Autodesk Inventor part; units mm, degrees
ref_plane "YZ Plane" through (0, 0, 0) normal (1, 0, 0) x (0, 1, 0)
ref_plane "XZ Plane" through (0, 0, 0) normal (0, 1, 0) x (-1, 0, 0)
ref_plane "XY Plane" through (0, 0, 0) normal (0, 0, 1) x (1, 0, 0)
sketch "Sketch1" plane through (0, 0, 0) normal (0, 1, 0) x (-1, 0, 0)
  circle A0 centre (0, 0) radius 9.625
  circle A1 centre (0, 0) radius 7.7
  dimension "d0" = 19.25
  dimension "d1" = 15.4
extrude "Extrusion1" add sketch "Sketch1" along normal blind 1
sketch "Sketch2" plane through (0, 1, 0) normal (0, 1, 0) x (1, 0, 0)
  circle A0 centre (0, 0) radius 9.6436
  line L0 (-2.8579, 4.95) -> (2.8579, 4.95)
  line L1 (2.8579, 4.95) -> (5.7158, 0)
  line L2 (5.7158, 0) -> (2.8579, -4.95)
  line L3 (2.8579, -4.95) -> (-2.8579, -4.95)
  line L4 (-2.8579, -4.95) -> (-5.7158, 0)
  line L5 (-5.7158, 0) -> (-2.8579, 4.95)
  line L6 (0, 0) -> (0, -3.104)
  line L7 (0, 0) -> (3.104, 0) construction
  dimension "d4" = 9.9
  dimension "d5" = 90
extrude "Extrusion2" add sketch "Sketch2" along normal blind 6
sketch "Sketch3" plane through (0, 7, 0) normal (0, 1, 0) x (1, 0, 0)
  circle A0 centre (0, 0) radius 9.6436
  circle A1 centre (0, 0) radius 2.75
  circle A2 centre (0, 0) radius 9.6436
  dimension "d8" = 5.5
  dimension "d9" = 0
extrude "Extrusion3" add sketch "Sketch3" along normal blind 1
fillet "Fillet1" radius 0.2 2 edges at (9.625, 0, 0) (7.7, 0, 0)
properties part number "NutRetainer"
Read the model definition and answer for the solid it produces. Units are mm, in the model's axes. A direction names the side the tool comes from. Give positions to 0.01 mm unless a question says otherwise; leave off trailing zeros. Loops run counter-clockwise (first coordinate to the right, second up) from the corner with the lowest first, then second, coordinate; pieces in that order, holes last. Notation, with made-up numbers: (-14.75, 77) - (-2.75, 77) arc R31 ccw to (-2.75, 102) - close; hole circle Ø4 at (74, -16.5). An arc over 180 degrees is marked (long way). Answer as CSV lines item,"result". Start each with the question number.
1) Which of the six approach directions +Z, -Z, +X, -X, +Y, -Y give full straight-line access (tool end or side, diameter ignored) to faces 5 (the face through (4.267, 3.958, -2.51)), 6 (the face through (-2.3, 8, 2))?
2) Find section B-B (y = 6). Write down the section's boundary in (x, z).
3) Determine the mould class of faces 1 (the face through (4.307, 3.958, 2.44)), 2 (the face through (0, 4, -4.95)), 3 (the face through (2, 0, -8)), 4 (the face through (7.638, 0.594, 5.857)) for opening direction Z: released by +Z, released by -Z, zero draft, split by the parting line, or undercut.
4) Each of these flat-tipped pins is pushed along its axis until it touches: pin 1 Ø3 at (x, y) = (-3, 2.5) entering from +Z; pin 2 Ø8 at (x, z) = (0, -0.5) entering from -Y; pin 3 Ø3 at (x, y) = (3, 2.5) entering from -Z; pin 4 Ø6.5 at (x, z) = (0, 0) entering from +Y. Where does it stop, or does it pass through?
5) Straight lines are drawn through the part: L1, parallel to X at y = 7.2, z = 0; L2, parallel to Z at x = 0, y = 0.85 (3 decimals). For each, find the intervals that lie inside material, in ascending order. Write a range as from..to.
6) Find section A-A (x = 0). Write down the section's boundary in (y, z) (3 decimals), then the cut area to 3 significant figures.
Findings below:
1,face 5,"-Y"
1,face 6,"+Z, -Z, +X, -X, +Y"
2,outline,"circle Ø19.29 at (0, 0); hole (-5.72, 0) - (-2.86, -4.95) - (2.86, -4.95) - (5.72, 0) - (2.86, 4.95) - (-2.86, 4.95) - close"
3,face 1,"undercut"
3,face 2,"undercut"
3,face 3,"zero draft"
3,face 4,"split by the parting line"
4,pin 1,"z = 9.53"
4,pin 2,"y = 7"
4,pin 3,"z = -9.53"
4,pin 4,"y = 8"
5,L1,"-9.64..-2.75, 2.75..9.64"
5,L2,"-9.625..-7.7, 7.7..9.625"
6,outline,"(0, -9.425) arc R0.2 ccw to (0.2, -9.625) - (1, -9.625) - (1, -9.644) - (8, -9.644) - (8, -2.75) - (7, -2.75) - (7, -4.95) - (1, -4.95) - (1, -7.7) - (0.2, -7.7) arc R0.2 ccw to (0, -7.9) - close; (0, 7.9) arc R0.2 ccw to (0.2, 7.7) - (1, 7.7) - (1, 4.95) - (7, 4.95) - (7, 2.75) - (8, 2.75) - (8, 9.644) - (1, 9.644) - (1, 9.625) - (0.2, 9.625) arc R0.2 ccw to (0, 9.425) - close"
6,area,"73.9 mm^2"
